Check sheet for the drawn part. Datum: minimum x, y, z corner. Units: mm. Round coordinates to 2 decimals unless told otherwise and drop trailing zeros. Order: outer loops, then holes, each group sorted by start corner. A loop starts at its lowest first (then second) coordinate and runs counter-clockwise, first axis right, second up.
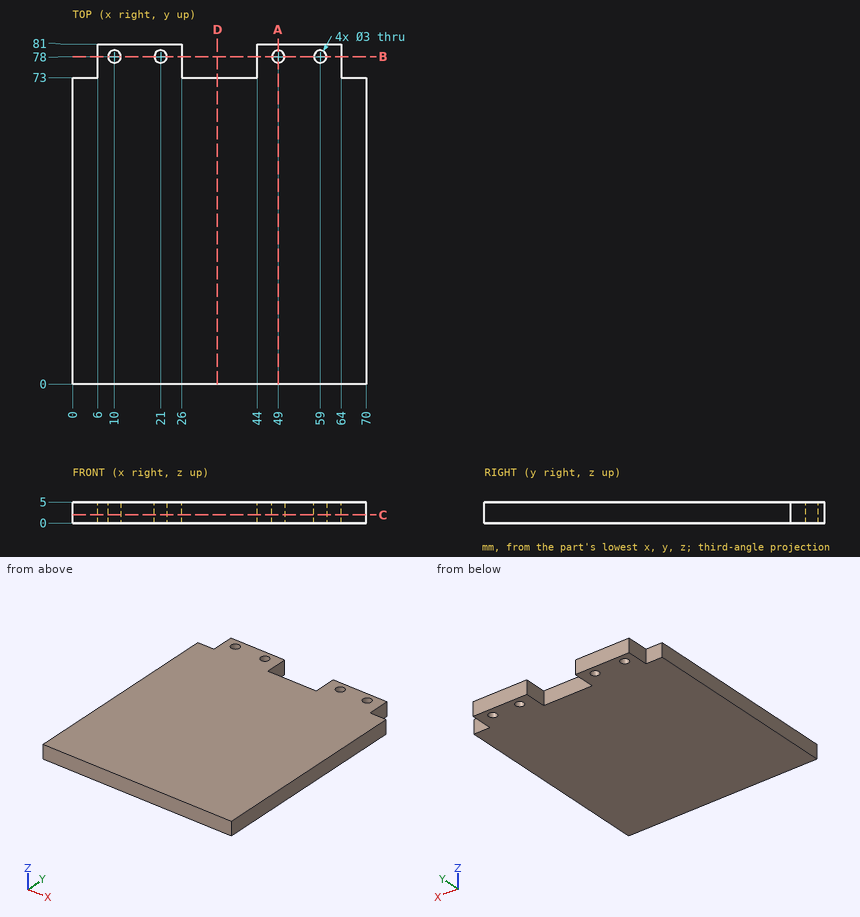
(1) Sectioned sample at A-A, the plane x = 49. Record the cut outline in (y, z).
Returned:
outline: (0, 0) - (76.5, 0) - (76.5, 5) - (0, 5) - close; (79.5, 0) - (81, 0) - (81, 5) - (79.5, 5) - close
(2) Sectioned sample at C-C, the plane z = 1.95. Record the cut outline in (x, y), and give its area (3 significant figures).
Returned:
outline: (0, 0) - (70, 0) - (70, 73) - (64, 73) - (64, 81) - (44, 81) - (44, 73) - (26, 73) - (26, 81) - (6, 81) - (6, 73) - (0, 73) - close; hole circle Ø3 at (10, 78); hole circle Ø3 at (21, 78); hole circle Ø3 at (49, 78); hole circle Ø3 at (59, 78)
area: 5,400 mm2
(3) Sectioned sample at B-B, the plane y = 78. Record the cut outline in (x, z), and give its area (3 significant figures).
Returned:
outline: (6, 0) - (8.5, 0) - (8.5, 5) - (6, 5) - close; (11.5, 0) - (19.5, 0) - (19.5, 5) - (11.5, 5) - close; (22.5, 0) - (26, 0) - (26, 5) - (22.5, 5) - close; (44, 0) - (47.5, 0) - (47.5, 5) - (44, 5) - close; (50.5, 0) - (57.5, 0) - (57.5, 5) - (50.5, 5) - close; (60.5, 0) - (64, 0) - (64, 5) - (60.5, 5) - close
area: 140 mm2
(4) Material ranges on line 1 (X direction, y = 78, z = 2.15); line 2 (Y direction, x = 10, z = 2.65); line 3 (Y direction, x = 5, z = 1.4), recorded low to high.
Returned:
line 1: x = 6 to 8.5, 11.5 to 19.5, 22.5 to 26, 44 to 47.5, 50.5 to 57.5, 60.5 to 64
line 2: y = 0 to 76.5, 79.5 to 81
line 3: y = 0 to 73
(5) Depth check by flat-ended pin: P1, Ø5, axis at x = 49, y = 78, coming from the +Z side; P2, Ø2.5, axis at y = 76, z = 3, coming from the -X side; P3, Ø2.5, axis at x = 66.5, z = 3.5, coming from the +Y side; P4, Ø1.8, axis at x = 59, y = 78, coming from the +Z side. Enter the tip coordinate at first touch or a pass-through.
Returned:
P1: stops at z = 5
P2: stops at x = 6
P3: stops at y = 73
P4: passes through
(6) Sectioned sample at D-D, the plane x = 34.5. Record the cut outline in (y, z).
Returned:
outline: (0, 0) - (73, 0) - (73, 5) - (0, 5) - close
